Check sheet for the drawn part. Datum: minimum x, y, z corner. Units: mm. Round coordinates to 2 decimals unless told otherwise and drop trailing zeros. Write each loop counter-clockwise with the first axis right and the second up, starting at its lowest first coordinate (ties: lowest second). Pieces come first, ordered by that corner, then holes. Notation, with made-up numbers: (39, 45.25) - (56, 45.25) arc R8 ccw to (56, 50.25) - close; hole circle Ø7 at (58.25, 77). An arc over 180 degrees is marked (long way). Write each question's results on one line, items separated by ' | '.
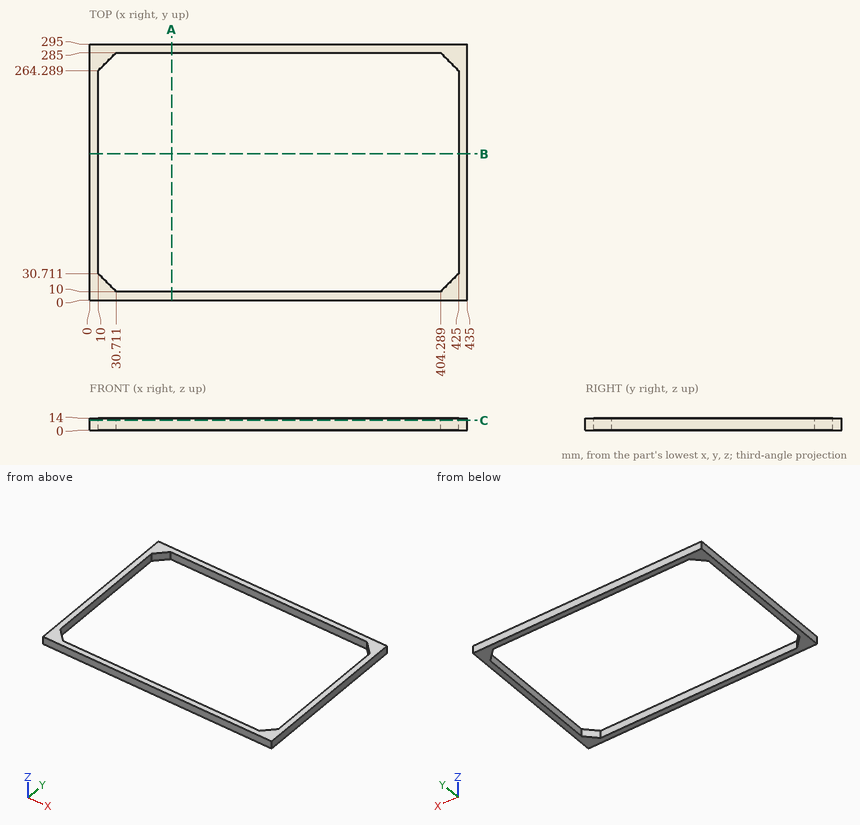
(1) Section check A-A (x = 94.5). Record the cut outline in (y, z), plus the area to 3 significant figures.
Answer:
outline: (0, 0) - (10, 0) - (10, 14) - (0, 14) - close; (285, 0) - (295, 0) - (295, 14) - (285, 14) - close | area: 280 mm2
(2) Section check B-B (y = 168.5). Record the cut outline in (x, z).
Answer:
outline: (0, 0) - (10, 0) - (10, 14) - (0, 14) - close; (425, 0) - (435, 0) - (435, 14) - (425, 14) - close
(3) Section check C-C (z = 11.5). Record the cut outline in (x, y), plus the area to 3 significant figures.
Answer:
outline: (0, 0) - (435, 0) - (435, 295) - (0, 295) - close; hole (10, 30.71) - (30.71, 10) - (404.29, 10) - (425, 30.71) - (425, 264.29) - (404.29, 285) - (30.71, 285) - (10, 264.29) - close | area: 15,100 mm2
(4) Thickness scan on L1, parallel to Y at x = 279, z = 11.5; L2, parallel to X at y = 75.5, z = 11.5; L3, parallel to X at y = 17, z = 6.5. Record the ranges inside material, lowest first.
Answer:
L1: 0 to 10, 285 to 295 | L2: 0 to 10, 425 to 435 | L3: 0 to 23.71, 411.29 to 435
